from build123d import *

# Parameters (mm, degrees)
ESQUISSE1_R             = 2
BOSS_EXTRU_1_DEPTH      = 6
CONG_1_R                = 10
CONG_2_R                = 5
CHANFREIN1_SIZE         = 2
ESQUISSE2_R             = 1.1
ENL_V_MAT_EXTRU_1_DEPTH = 6


with BuildPart() as part:
    # Esquisse1 → Boss.-Extru.1 (new body)
    with BuildSketch(Plane.XY):
        Polygon((-36.081854409, 9.183471646), (-36.081854409, -28.816528354), (16.168145591, -28.816528354), (16.168145591, -19.816528354), (-6.081854409, -19.816528354), (-6.081854409, 0.183471646), (16.168145591, 0.183471646), (16.168145591, 9.183471646), align=None)
        with Locations((-26.081854409, 0.183471646)):
            Circle(ESQUISSE1_R, mode=Mode.SUBTRACT)
        with Locations((-26.081854409, -19.816528354)):
            Circle(ESQUISSE1_R, mode=Mode.SUBTRACT)
    extrude(amount=BOSS_EXTRU_1_DEPTH)

    # Congé1
    cong_1_edges = [part.edges().sort_by_distance(p)[0] for p in [
        (-36.081854409, -28.816528354, 3),
        (-36.081854409, 9.183471646, 3),
    ]]
    fillet(cong_1_edges, radius=CONG_1_R)

    # Congé2
    cong_2_edges = [part.edges().sort_by_distance(p)[0] for p in [
        (16.168145591, 9.183471646, 3),
        (16.168145591, -28.816528354, 3),
    ]]
    fillet(cong_2_edges, radius=CONG_2_R)

    # Chanfrein1
    chanfrein1_edges = [part.edges().sort_by_distance(p)[0] for p in [
        (16.168145591, 0.183471646, 3),
        (16.168145591, -19.816528354, 3),
    ]]
    chamfer(chanfrein1_edges, length=CHANFREIN1_SIZE)

    # Esquisse2 → Enlèv. mat.-Extru.1 (cut)
    with BuildSketch(Plane.XY.offset(6)):
        with Locations((-4.081854409, 3.683471646)):
            Circle(ESQUISSE2_R)
        with Locations((3.918145591, 3.683471646)):
            Circle(ESQUISSE2_R)
        with Locations((11.918145591, 3.683471646)):
            Circle(ESQUISSE2_R)
        with Locations((-9.581854409, -1.816528354)):
            Circle(ESQUISSE2_R)
        with Locations((-9.581854409, -17.816528354)):
            Circle(ESQUISSE2_R)
        with Locations((-4.081854409, -23.316528354)):
            Circle(ESQUISSE2_R)
        with Locations((3.918145591, -23.316528354)):
            Circle(ESQUISSE2_R)
        with Locations((11.918145591, -23.316528354)):
            Circle(ESQUISSE2_R)
    extrude(amount=-ENL_V_MAT_EXTRU_1_DEPTH, mode=Mode.SUBTRACT)


solid = part.part
Check sheet for the modelled part. Datum: model origin and axes. Units: mm. A direction names the side the tool comes from. Round coordinates to 2 decimals unless told otherwise and drop trailing zeros. Loops run counter-clockwise (first coordinate to the right, second up) from the corner with the lowest first, then second, coordinate; pieces in that order, holes last. Notation, with made-up numbers: M -17,49.25 L 4,49.25 A22 cw 4,72.25 Z; hole C 81.25,42 d11. An arc over 180 degrees is marked long. One line per question, with ' | ' between items. Start each with the question number.
Item 1: Set-up check for faces 1 (the face through (15.18, -20.83, 2.96)), 2 (the face through (-36.082, -10, 3)): record each of +Z, -Z, +X, -X, +Y, -Y from which the full face is reachable in a straight line by a thin tool's end or side.
Item 2: Section check D-D (x = -30). Record the boundary of the cut face in (y, z).
Item 3: Section check C-C (y = -10). Record the boundary of the cut face in (x, z).
Item 4: Scan lines: probe 1 along Y at (x, z) = (-4, 4.8); probe 2 along Y at (x, z) = (-6, 3.05); probe 3 along Y at (x, z) = (12, 1.2). Record each from-to range of solid material in increasing order.
Item 5: Section check A-A (x = -1). Record the boundary of the cut face in (y, z).
Item 6: Section check B-B (z = 3.3). State how many separate pieces and enclosed holes the cut face has, and give its area (3 significant figures).
Item 7: Release check for a two-part mould opening along Y. For faces 3 (the face through (-28.08, 0.27, 2.96)), 4 (the face through (14.66, 7.76, 3.04)), 5 (the face through (-16, -10, 0)) record: released by +Y, released by -Y, zero draft, split by the parting line, or undercut.
Worked out:
1) face 1: +Z, -Z, +X | face 2: +Z, -Z, -X, +Y, -Y
2) outline: M -28.02,0 L 8.38,0 L 8.38,6 L -28.02,6 Z
3) outline: M -36.08,0 L -6.08,0 L -6.08,6 L -36.08,6 Z
4) probe 1: -28.82 to -24.41, -22.22 to -19.82, 0.18 to 2.59, 4.78 to 9.18 | probe 2: -28.82 to -19.82, 0.18 to 9.18 | probe 3: -28.75 to -24.41, -22.22 to -19.82, 0.18 to 2.59, 4.78 to 9.11
5) outline: M -28.82,0 L -19.82,0 L -19.82,6 L -28.82,6 Z; M 0.18,0 L 9.18,0 L 9.18,6 L 0.18,6 Z
6) separate pieces: 1 | enclosed holes: 10 | area: 1,430 mm^2
7) face 3: undercut | face 4: released by +Y | face 5: zero draft
